from build123d import *

# Parameters (mm, degrees)
F1_DEPTH = 32.5
F2_R     = 5


with BuildPart() as f1:
    # F0 (on Top) → F1 (new body, symmetric)
    with BuildSketch(Plane.XY):
        with BuildLine():
            Line((0, -5.344), (0, 12.356))
            Line((0, 12.356), (-49, 12.356))
            ThreePointArc((-49, 12.356), (-49.707107, 12.063107), (-50, 11.356))
            Line((-50, 11.356), (-50, 10.356))
            ThreePointArc((-50, 10.356), (-49.707107, 9.648893), (-49, 9.356))
            Line((-49, 9.356), (-48.25, 9.356))
            ThreePointArc((-48.25, 9.356), (-47.542893, 9.648893), (-47.25, 10.356))
            Line((-47.25, 10.356), (-43, 10.356))
            Line((-43, 10.356), (-43, 7.656))
            ThreePointArc((-43, 7.656), (-42.707107, 6.948893), (-42, 6.656))
            Line((-42, 6.656), (-10, 6.656))
            Line((-10, 6.656), (-10, -2.344))
            Line((-10, -2.344), (-49, -2.344))
            ThreePointArc((-49, -2.344), (-49.707107, -2.636893), (-50, -3.344))
            Line((-50, -3.344), (-50, -4.344))
            ThreePointArc((-50, -4.344), (-49.707107, -5.051107), (-49, -5.344))
            Line((-49, -5.344), (0, -5.344))
        make_face()
    extrude(amount=F1_DEPTH, both=True)

    # F2
    f2_edges = [f1.edges().sort_by_distance(p)[0] for p in [
        (0, 3.506, 32.5),
        (0, 3.506, -32.5),
    ]]
    fillet(f2_edges, radius=F2_R)


solid = f1.part
Source: CAD feature listing. Evaluate the final solid. Frame: model axes, mm. A direction names the side the tool comes from. Round coordinates to 2 decimals unless told otherwise and drop trailing zeros. Write each loop counter-clockwise with the first axis right and the second up, starting at its lowest first coordinate (ties: lowest second). Pieces come first, ordered by that corner, then holes. Notation, with made-up numbers: M 59.5,7 L 104.5,7 A32 cw 104.5,42 Z; hole C 8.5,13.5 d4. An arc over 180 degrees is marked long. One line per item, written item: value. Start each with the question number.
Item 1: Pin query (flat end, axial travel): pin 1 (2 mm diameter, centred on y = 9, z = -2.5, fed in from -X); pin 2 (8 mm diameter, centred on y = 2, z = 26, fed in from -X). Return the tip coordinate at first contact, or that it passes through.
Item 2: Section query D-D (y = 1.75). Return the cut outline in (x, z).
Item 3: Set-up query: faces 1 (the flat face through (-10, 2, 0)), 2 (the flat face through (-43, 9, 0)), 3 (the cylindrical face through (-1.43, 3.63, -31)). Return all of +Z, -Z, +X, -X, +Y, -Y with unobstructed straight access to the full face (end or side cutting, diameter ignored); none if empty.
Item 4: Section query C-C (x = -11). Return the cut outline in (y, z).
Item 5: Section query A-A (x = -46). Return the cut outline in (y, z), plus the area to 3 significant figures.
Item 6: Section query B-B (z = 21.5). Return the cut outline in (x, y), plus the area to 3 significant figures.
Item 7: Ray query, L1, parallel to Y at x = -12.5, z = -21; L2, parallel to X at y = -0.5, z = 1; L3, parallel to X at y = -3.25, z = 15. Return the intervals inside material, ascending. Write a range as from..to.
Item 8: Mould query, pull axis Y, two halves, no side actions, for faces 4 (the flat face through (0, 3, 0)), 5 (the flat face through (-45, 10.356, 0)), 6 (the flat face through (-24, 12.356, 0)). Classes: pulls with the +Y half, pulls with the -Y half, needs draft (parallel to the pull), parting line crosses it, or undercut.
Result set:
1. pin 1: stops at x = -49.93
1. pin 2: stops at x = -10
2. outline: M -10,-32.5 L -5,-32.5 A5 ccw 0,-27.5 L 0,27.5 A5 ccw -5,32.5 L -10,32.5 Z
3. face 1: +Z, -Z, -X
3. face 2: +Z, -Z
3. face 3: -Z, +X, +Y, -Y
4. outline: M -5.34,-32.5 L -2.34,-32.5 L -2.34,32.5 L -5.34,32.5 Z; M 6.66,-32.5 L 12.36,-32.5 L 12.36,32.5 L 6.66,32.5 Z
5. outline: M -5.34,-32.5 L -2.34,-32.5 L -2.34,32.5 L -5.34,32.5 Z; M 10.36,-32.5 L 12.36,-32.5 L 12.36,32.5 L 10.36,32.5 Z
5. area: 325 mm²
6. outline: M -50,-4.34 A1 ccw -49,-5.34 L 0,-5.34 L 0,12.36 L -49,12.36 A1 ccw -50,11.36 L -50,10.36 A1 ccw -49,9.36 L -48.25,9.36 A1 ccw -47.25,10.36 L -43,10.36 L -43,7.66 A1 ccw -42,6.66 L -10,6.66 L -10,-2.34 L -49,-2.34 A1 ccw -50,-3.34 Z
6. area: 501 mm²
7. L1: y = -5.34..-2.34, 6.66..12.36
7. L2: x = -10..0
7. L3: x = -50..0
8. face 4: needs draft
8. face 5: undercut
8. face 6: pulls with the +Y half
